Can you work these out from the model? Positions are in its coordinate system, mm. A direction names the side the tool comes from. Give positions to 0.01 mm unless a question says otherwise; leave off trailing zeros. Write each loop counter-clockwise with the first axis right and the second up, starting at its lowest first coordinate (ties: lowest second). Pieces come first, ordered by that corner, then holes. Notation, with made-up numbers: (-4, 48) -> (13, 48) arc R10 ccw to (13, 57) -> close; hole circle Ø3 at (6.25, -25.5). An arc over 180 degrees is marked (long way). One line per item, written item: value.
from build123d import *

# Parameters (mm, degrees)
F0_W         = 100
F0_H         = 100
F1_DEPTH     = 100
F2_T         = -10
F3_W         = 80
F3_H         = 10
F4_DEPTH     = 100
F6_W         = 100
F6_H         = 100
F7_DEPTH     = 25
F8_R         = 10
F9_R         = 10
F10_T1_DEPTH = 90
F10_S5_W     = 10
F10_S5_H     = 10
F10_T6_DEPTH = 10
F11_T1_DEPTH = 15
F11_S5_W     = 10.2
F11_S5_H     = 10.2
F11_T6_DEPTH = 10.2


# Not quite as in the source:
# - a fillet or chamfer that OpenCascade refuses, or shapes differently, is made with other operations: its cross-section is extruded or revolved along the edge and cut away or added


with BuildPart() as f1:
    # F0 (on Top) → F1 (new body)
    with BuildSketch(Plane.XY):
        Rectangle(F0_W, F0_H)
    extrude(amount=F1_DEPTH)

    # F2
    f2_openings = [f1.faces().sort_by_distance(p)[0] for p in [
        (0, 0, 100),
    ]]
    offset(amount=F2_T, openings=f2_openings)

    # F3 (on Top) → F4 (join)
    with BuildSketch(Plane.XY):
        Rectangle(F3_W, F3_H)
    extrude(amount=F4_DEPTH)

    # F6 (on offset) → F7 (join)
    with BuildSketch(Plane.XY.offset(100)):
        with Locations((0.513449031, 0.0360049307)):
            Rectangle(F6_W, F6_H)
    extrude(amount=F7_DEPTH)

    # F8
    f8_edges = [f1.edges().sort_by_distance(p)[0] for p in [
        (0.513449, 50.036005, 125),
        (-49.486551, 0.036005, 125),
        (0.513449, -49.963995, 125),
        (50.513449, 0.036005, 125),
    ]]
    fillet(f8_edges, radius=F8_R)

    # F9
    f9_edges = [f1.edges().sort_by_distance(p)[0] for p in [
        (0, -50, 0),
        (50, 0, 0),
        (0, 50, 0),
        (-50, 0, 0),
    ]]
    fillet(f9_edges, radius=F9_R)

    # F10: fillet of radius 10 on 1 edges, made by hand

    # F10_s2 → F10_t1 (cut)
    with BuildSketch(Plane.XY.offset(10)):
        with BuildLine():
            ThreePointArc((50, -40), (47.0710678119, -47.0710678119), (40, -50))
            Line((40, -50), (50, -50))
            Line((50, -50), (50, -40))
        make_face()
    extrude(amount=F10_T1_DEPTH, mode=Mode.SUBTRACT)


with BuildPart() as f10_tool4:
    # F10_s5 → F10_t6 (new body)
    with BuildSketch(Plane.YZ.offset(40)):
        with Locations((-45, 5)):
            Rectangle(F10_S5_W, F10_S5_H)
    extrude(amount=F10_T6_DEPTH)

    # F10_s7 → F10_t8 (revolve, cut)
    with BuildSketch(Plane(origin=(40, -40, 10), x_dir=(0, 0.7071067812, 0.7071067812), z_dir=(0, 0.7071067812, -0.7071067812))):
        with BuildLine():
            ThreePointArc((0, -10), (10, 0), (0, 10))
            Line((0, 10), (0, -10))
        make_face()
    revolve(axis=Axis((40, -40, 10), (1, 0, 0)), mode=Mode.SUBTRACT)


with BuildPart() as f1_1:
    add(f1.part)

    # F10_t3: cut F10_tool4
    add(f10_tool4.part, mode=Mode.SUBTRACT)

    # F11: fillet of radius 10 on 1 edges, made by hand

    # F11_s2 → F11_t1 (cut)
    with BuildSketch(Plane.XY.offset(100)):
        with BuildLine():
            ThreePointArc((50.513449031, -39.9639950693), (47.5845168429, -47.0350628811), (40.513449031, -49.9639950693))
            Line((40.513449031, -49.9639950693), (50.513449031, -49.9639950693))
            Line((50.513449031, -49.9639950693), (50.513449031, -39.9639950693))
        make_face()
    extrude(amount=F11_T1_DEPTH, mode=Mode.SUBTRACT)


with BuildPart() as f11_tool4:
    # F11_s5 → F11_t6 (new body)
    with BuildSketch(Plane.YZ.offset(40.513449031)):
        with Locations((-45.0639950693, 120.1)):
            Rectangle(F11_S5_W, F11_S5_H)
    extrude(amount=F11_T6_DEPTH)

    # F11_s7 → F11_t8 (revolve, cut)
    with BuildSketch(Plane(origin=(40.513449031, -39.9639950693, 115), x_dir=(0, 0.7071067812, -0.7071067812), z_dir=(0, -0.7071067812, -0.7071067812))):
        with BuildLine():
            ThreePointArc((0, -10), (10, 0), (0, 10))
            Line((0, 10), (0, -10))
        make_face()
    revolve(axis=Axis((40.513449031, -39.9639950693, 115), (1, 0, 0)), mode=Mode.SUBTRACT)


with BuildPart() as f1_2:
    add(f1_1.part)

    # F11_t3: cut F11_tool4
    add(f11_tool4.part, mode=Mode.SUBTRACT)


solid = f1_2.part
1) If we section it at C-C (y = -31.5): Write out the boundary of the cut face in (x, z).
Answer list:
outline: (-50, 10) arc R10 ccw to (-40, 0) -> (40, 0) arc R10 ccw to (50, 10) -> (50, 100) -> (50.51, 100) -> (50.51, 115) arc R10 ccw to (40.51, 125) -> (-39.49, 125) arc R10 ccw to (-49.49, 115) -> (-49.49, 100) -> (-50, 100) -> close; hole (-40, 10) -> (40, 10) -> (40, 100) -> (-40, 100) -> close
2) Will these pins go through, and if not, where does the flat tip stop? pin 1 (12 mm diameter, centred on x = 1, z = 109, fed in from -Y); pin 2 (1 mm diameter, centred on x = 19, z = 14, fed in from +Y); pin 3 (1.5 mm diameter, centred on y = -9, z = 45, fed in from +X).
Answer list:
pin 1: stops at y = -49.96
pin 2: stops at y = 50
pin 3: stops at x = 50
3) If we section it at B-B (x = -1): State how many separate pieces and enclosed holes the cut face has, and give its area (3 significant figures).
Answer list:
separate pieces: 1
enclosed holes: 2
area: 6,110 mm^2
4) For faces 1 (the face through (-4.37, -47.15, 3.01)), 2 (the face through (-49.487, -1, 107)), 3 (the face through (50, 4, 54)), 4 (the face through (-1, -40, 54)), which set-ups out of +Z, -Z, +X, -X, +Y, -Y let a thin tool reach every point of the face, with its end or its side?
Answer list:
face 1: -Z, +X, -X, -Y
face 2: +Z, -X, +Y, -Y
face 3: -Z, +X, +Y, -Y
face 4: none
5) I need wall thicknesses on L1, parallel to Y at x = -7, z = 41; L2, parallel to X at y = -17, z = 63; L3, parallel to Z at x = -34, y = -13. Which ranges of each line are inside material? Lowest first, please.
Answer list:
L1: y = -50 to -40, -5 to 5, 40 to 50
L2: x = -50 to -40, 40 to 50
L3: z = 0 to 10, 100 to 125
6) We'd pull the mould along X, two halves only. Please class faces 5 (the face through (-1, -22, 100)), 6 (the face through (-5, -49.964, 107)), 7 (the face through (50.513, 4, 107)), 8 (the face through (-47.15, 0.7, 3.01)): released by +X, released by -X, zero draft, split by the parting line, or undercut.
Answer list:
face 5: undercut
face 6: zero draft
face 7: released by +X
face 8: released by -X
7) If we section it at A-A (z = 61): Write out the boundary of the cut face in (x, y).
Answer list:
outline: (-50, -50) -> (40, -50) arc R10 ccw to (50, -40) -> (50, 50) -> (-50, 50) -> close; hole (-40, -40) -> (40, -40) -> (40, -5) -> (-40, -5) -> close; hole (-40, 5) -> (40, 5) -> (40, 40) -> (-40, 40) -> close
